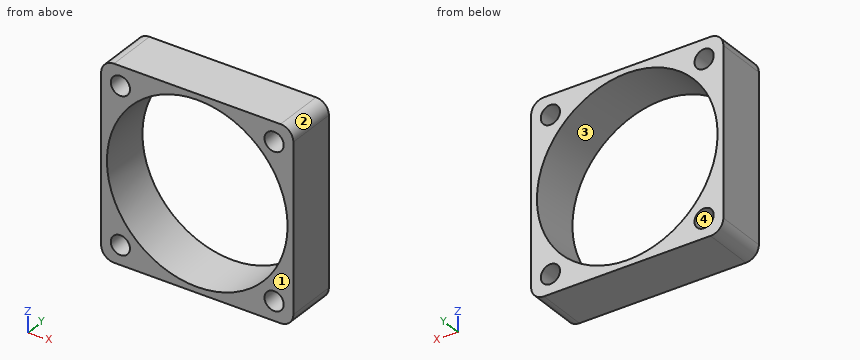
```python
from build123d import *

# Parameters (mm, degrees)
SKETCH1_W           = 30
SKETCH1_H           = 30
BOSS_EXTRUDE1_DEPTH = 8
FILLET1_R           = 2
SKETCH2_R           = 1.5
CUT_EXTRUDE1_DEPTH  = 8
SKETCH3_R           = 14.1
CUT_EXTRUDE2_DEPTH  = 8


with BuildPart() as part:
    # Sketch1 → Boss-Extrude1 (new body)
    with BuildSketch(Plane(origin=(0, 0, 0), x_dir=(1, 0, 0), z_dir=(0, 1, 0))):
        Rectangle(SKETCH1_W, SKETCH1_H)
    extrude(amount=BOSS_EXTRUDE1_DEPTH)

    # Fillet1
    fillet1_edges = [part.edges().sort_by_distance(p)[0] for p in [
        (-15, 4, -15),
        (15, 4, -15),
        (15, 4, 15),
        (-15, 4, 15),
    ]]
    fillet(fillet1_edges, radius=FILLET1_R)

    # Sketch2 → Cut-Extrude1 (cut)
    with BuildSketch(Plane(origin=(0, 8, 0), x_dir=(1, 0, 0), z_dir=(0, 1, 0))):
        with Locations((-12, 12)):
            Circle(SKETCH2_R)
        with Locations((12, 12)):
            Circle(SKETCH2_R)
        with Locations((-12, -12)):
            Circle(SKETCH2_R)
        with Locations((12, -12)):
            Circle(SKETCH2_R)
    extrude(amount=-CUT_EXTRUDE1_DEPTH, mode=Mode.SUBTRACT)

    # Sketch3 → Cut-Extrude2 (cut)
    with BuildSketch(Plane(origin=(0, 8, 0), x_dir=(1, 0, 0), z_dir=(0, 1, 0))):
        Circle(SKETCH3_R)
    extrude(amount=-CUT_EXTRUDE2_DEPTH, mode=Mode.SUBTRACT)


solid = part.part
```
Here's how the part is built. I have some questions about the finished solid (model axes, mm). Face numbers are marked on the shaded views. Round coordinates to 2 decimals unless told otherwise and drop trailing zeros. Loops run counter-clockwise (first coordinate to the right, second up) from the corner with the lowest first, then second, coordinate; pieces in that order, holes last.
1. If I drill on probe 1 along X at (y, z) = (5.5, -12); probe 2 along X at (y, z) = (2.5, 12.5), over which ranges is the centre line in solid material (lowest first)?
Answers:
probe 1: x = -15 to -13.5, -10.5 to -7.4, 7.4 to 10.5, 13.5 to 15
probe 2: x = -15 to -13.41, -10.59 to -6.52, 6.52 to 10.59, 13.41 to 15
2. Suppose I cut it at A-A, the plane z = 0. Please give me the cut outline in (x, y), and give its area (3 significant figures).
Answers:
outline: (-15, 0) - (-14.1, 0) - (-14.1, 8) - (-15, 8) - close; (14.1, 0) - (15, 0) - (15, 8) - (14.1, 8) - close
area: 14.4 mm2
3. Suppose I cut it at C-C, the plane z = 12. Please give me the cut outline in (x, y).
Answers:
outline: (-15, 0) - (-13.5, 0) - (-13.5, 8) - (-15, 8) - close; (-10.5, 0) - (-7.4, 0) - (-7.4, 8) - (-10.5, 8) - close; (7.4, 0) - (10.5, 0) - (10.5, 8) - (7.4, 8) - close; (13.5, 0) - (15, 0) - (15, 8) - (13.5, 8) - close
4. Thinking about a two-plate mould opening in Z: for the marked faces 1, 2, 3 and 4, which applies, released by +Z, released by -Z, zero draft, split by the parting line, or undercut?
Answers:
face 1: zero draft
face 2: released by +Z
face 3: undercut
face 4: undercut
5. Suppose I cut it at B-B, the plane x = 0. Please give me the cut outline in (y, z), and give its area (3 significant figures).
Answers:
outline: (0, -15) - (8, -15) - (8, -14.1) - (0, -14.1) - close; (0, 14.1) - (8, 14.1) - (8, 15) - (0, 15) - close
area: 14.4 mm2
6. Will these pins go through, and if not, where does the flat tip stop? pin 1 (3 mm diameter, centred on x = -8, z = 10, fed in from +Y); pin 2 (2.5 mm diameter, centred on x = -12, z = -12, fed in from -Y) (1 decimal).
Answers:
pin 1: stops at y = 8
pin 2: passes through
7. Suppose I cut it at D-D, the plane y = 1. Please give me the cut outline in (x, z), and give its area (3 significant figures).
Answers:
outline: (-15, -13) arc R2 ccw to (-13, -15) - (13, -15) arc R2 ccw to (15, -13) - (15, 13) arc R2 ccw to (13, 15) - (-13, 15) arc R2 ccw to (-15, 13) - close; hole circle Ø28.2 at (0, 0); hole circle Ø3 at (-12, -12); hole circle Ø3 at (-12, 12); hole circle Ø3 at (12, -12); hole circle Ø3 at (12, 12)
area: 244 mm2
